Source: CAD feature listing. Evaluate the final solid. Frame: model axes, mm. A direction names the side the tool comes from. Coordinates: 2 decimals unless noted, no trailing zeros. Order: outer loops, then holes, each group sorted by start corner. A loop starts at its lowest first (then second) coordinate and runs counter-clockwise, first axis right, second up. Notation, with made-up numbers: (-37.75, 4.5) - (-15.75, 4.5) arc R34 ccw to (-15.75, 40.5) - close; hole circle Ø4 at (44.5, -28). An arc over 180 degrees is marked (long way). One line per question, with ' | ' between items.
from build123d import *

# Parameters (mm, degrees)
BOSS_EXTRUDE1_DEPTH      = 40
BOSS_EXTRUDE1_DEPTH_BACK = 10
SKETCH1_W                = 73
SKETCH1_H                = 3
SKETCH1_W_2              = 3
SKETCH1_H_2              = 10
SKETCH5_R                = 2.05
CUT_EXTRUDE2_DEPTH       = 5.1
CUT_EXTRUDE3_DEPTH       = 82
SKETCH9_W                = 50
SKETCH9_H                = 13
CUT_EXTRUDE4_DEPTH       = 0.5
CUT_EXTRUDE5_DEPTH       = 98.5
FILLET2_R                = 4
FILLET3_R                = 1


with BuildPart() as part:
    # Sketch1 → Boss-Extrude1 (new, two sides: drawn at the far end of the back side and taken through both)
    with BuildSketch(Plane.XY.offset(-BOSS_EXTRUDE1_DEPTH_BACK)):
        with Locations((0, -34)):
            Rectangle(SKETCH1_W, SKETCH1_H)
        with Locations((35, -40.5)):
            Rectangle(SKETCH1_W_2, SKETCH1_H_2)
        with Locations((-35, -40.5)):
            Rectangle(SKETCH1_W_2, SKETCH1_H_2)
    extrude(amount=BOSS_EXTRUDE1_DEPTH + BOSS_EXTRUDE1_DEPTH_BACK)

    # Sketch5 → Cut-Extrude2 (cut)
    with BuildSketch(Plane(origin=(0, -32.5, 0), x_dir=(1, 0, 0), z_dir=(0, 1, 0))):
        with Locations(Location((-19, 4, 0), (0, 0, 270))):
            Circle(SKETCH5_R)
        with Locations(Location((19, 4, 0), (0, 0, 270))):
            Circle(SKETCH5_R)
        with Locations(Location((19, -34, 0), (0, 0, 270))):
            Circle(SKETCH5_R)
        with Locations(Location((-19, -34, 0), (0, 0, 270))):
            Circle(SKETCH5_R)
        with BuildLine():
            Line((-31.5, -17), (-31.5, -13))
            ThreePointArc((-31.5, -13), (-30, -11.5), (-28.5, -13))
            Line((-28.5, -13), (-28.5, -17))
            ThreePointArc((-28.5, -17), (-30, -18.5), (-31.5, -17))
        make_face()
        with BuildLine():
            Line((31.5, -13), (31.5, -17))
            ThreePointArc((31.5, -17), (30, -18.5), (28.5, -17))
            Line((28.5, -17), (28.5, -13))
            ThreePointArc((28.5, -13), (30, -11.5), (31.5, -13))
        make_face()
    extrude(amount=-CUT_EXTRUDE2_DEPTH, mode=Mode.SUBTRACT)

    # Sketch8 → Cut-Extrude3 (cut)
    with BuildSketch(Plane.ZY.offset(36.5)):
        with BuildLine():
            Line((5.75, -38.4), (7.25, -38.4))
            ThreePointArc((7.25, -38.4), (8.85, -40), (7.25, -41.6))
            Line((7.25, -41.6), (5.75, -41.6))
            ThreePointArc((5.75, -41.6), (4.15, -40), (5.75, -38.4))
        make_face()
        with BuildLine():
            Line((24.25, -38.4), (22.75, -38.4))
            ThreePointArc((22.75, -38.4), (21.15, -40), (22.75, -41.6))
            Line((22.75, -41.6), (24.25, -41.6))
            ThreePointArc((24.25, -41.6), (25.85, -40), (24.25, -38.4))
        make_face()
    extrude(amount=-CUT_EXTRUDE3_DEPTH, mode=Mode.SUBTRACT)

    # Sketch9 → Cut-Extrude4 (cut)
    with BuildSketch(Plane.ZY.offset(36.5)):
        with Locations((15, -39)):
            Rectangle(SKETCH9_W, SKETCH9_H)
    cut_extrude4 = extrude(amount=-CUT_EXTRUDE4_DEPTH, mode=Mode.SUBTRACT)

    # Mirror1: Cut-Extrude4 across plane
    add(cut_extrude4.mirror(Plane(origin=(0, 0, 0), x_dir=(0, 0, 1), z_dir=(1, 0, 0))), mode=Mode.SUBTRACT)

    # Sketch10 → Cut-Extrude5 (cut)
    with BuildSketch(Plane(origin=(36, 0, 0), x_dir=(0, 0, -1), z_dir=(1, 0, 0))):
        with BuildLine():
            Line((-39.673112404, -45.5), (-40.667568966, -46.550213702))
            Line((-40.667568966, -46.550213702), (-44.63224415, -43))
            Line((-44.63224415, -43), (-42.018495325, -33.98072497))
            Line((-42.018495325, -33.98072497), (-39.463482429, -29.927945893))
            Line((-39.463482429, -29.927945893), (-37.524182533, -32.5))
            ThreePointArc((-37.524182533, -32.5), (-38.383444331, -36.355587887), (-39.532044935, -40.135085929))
            ThreePointArc((-39.532044935, -40.135085929), (-40.017082913, -42.806643803), (-39.673112404, -45.5))
        make_face()
    cut_extrude5 = extrude(amount=-CUT_EXTRUDE5_DEPTH, mode=Mode.SUBTRACT)

    # Fillet2
    # the kernel refuses this fillet: 4 mm, written as the material it takes off along each edge
    with BuildSketch(Plane(origin=(23.5, -45.5, -10), x_dir=(0, 1, 0), z_dir=(1, 0, 0)), Plane(origin=(-46, -45.5, -10), x_dir=(0, 1, 0), z_dir=(1, 0, 0))) as fillet2_piece_1:
        with BuildLine():
            CenterArc((FILLET2_R, FILLET2_R), FILLET2_R, 180, 90)
            Line((0, FILLET2_R), (-FILLET2_R * 0.02, FILLET2_R))
            Line((-FILLET2_R * 0.02, FILLET2_R), (-FILLET2_R * 0.02, -FILLET2_R * 0.02))
            Line((-FILLET2_R * 0.02, -FILLET2_R * 0.02), (FILLET2_R, -FILLET2_R * 0.02))
            Line((FILLET2_R, -FILLET2_R * 0.02), (FILLET2_R, 0))
        make_face()
    extrude(amount=22.5, mode=Mode.SUBTRACT)
    with BuildSketch(Plane(origin=(43.633505106, -45.5, 39.673112404), x_dir=(0, 0, -1), z_dir=(-1, 0, 0)), Plane(origin=(-25.866494894, -45.5, 39.673112404), x_dir=(0, 0, -1), z_dir=(-1, 0, 0))) as fillet2_piece_2:
        with BuildLine():
            CenterArc((3.053402042, -4), FILLET2_R, 90, 57.679694788)
            Line((-0.326887596, -1.861392518), (-0.394493388, -1.818620368))
            ThreePointArc((-0.394493388, -1.818620368), (-0.291841099, -0.908147826), (-0.076877032, 0.022134181))
            Line((-0.076877032, 0.022134181), (0, 0.08))
            Line((0, 0.08), (3.053402042, 0.08))
            Line((3.053402042, 0.08), (3.053402042, 0))
        make_face()
    extrude(amount=17.767010212, mode=Mode.SUBTRACT)

    # Mirror2: Cut-Extrude5 across plane
    add(cut_extrude5.mirror(Plane.XY.offset(15)), mode=Mode.SUBTRACT)

    # Fillet3
    # the kernel refuses this fillet: 1 mm, written as the material it takes off along each edge
    with BuildSketch(Plane(origin=(36, -43.040322305, -1.130093667), x_dir=(0, 0.32679600244698914, -0.9450949014700414), z_dir=(0, 0.9450949014700414, 0.32679600244698914))) as fillet3_piece_1:
        with BuildLine():
            CenterArc((8.890060939 - FILLET3_R, FILLET3_R), FILLET3_R, 270, 90)
            Line((8.890060939 - FILLET3_R, 0), (8.890060939 - FILLET3_R, -FILLET3_R * 0.02))
            Line((8.890060939 - FILLET3_R, -FILLET3_R * 0.02), (8.890060939 + FILLET3_R * 0.02, -FILLET3_R * 0.02))
            Line((8.890060939 + FILLET3_R * 0.02, -FILLET3_R * 0.02), (8.890060939 + FILLET3_R * 0.02, FILLET3_R))
            Line((8.890060939 + FILLET3_R * 0.02, FILLET3_R), (8.890060939, FILLET3_R))
        make_face()
    revolve(axis=Axis((36, -43.040322305, -1.130093667), (-1, 0, 0)), revolution_arc=51.275424055, mode=Mode.SUBTRACT)
    with BuildSketch(Plane(origin=(36, -43.040322305, 31.130093667), x_dir=(0, 0.32679600244698914, 0.9450949014700414), z_dir=(0, 0.9450949014700414, -0.32679600244698914))) as fillet3_piece_2:
        with BuildLine():
            CenterArc((8.890060939 - FILLET3_R, -FILLET3_R), FILLET3_R, 0, 90)
            Line((8.890060939 - FILLET3_R, 0), (8.890060939 - FILLET3_R, FILLET3_R * 0.02))
            Line((8.890060939 - FILLET3_R, FILLET3_R * 0.02), (8.890060939 + FILLET3_R * 0.02, FILLET3_R * 0.02))
            Line((8.890060939 + FILLET3_R * 0.02, FILLET3_R * 0.02), (8.890060939 + FILLET3_R * 0.02, -FILLET3_R))
            Line((8.890060939 + FILLET3_R * 0.02, -FILLET3_R), (8.890060939, -FILLET3_R))
        make_face()
    revolve(axis=Axis((36, -43.040322305, 31.130093667), (1, 0, 0)), revolution_arc=53.885597182, mode=Mode.SUBTRACT)
    with BuildSketch(Plane(origin=(-36, -43.040322305, -1.130093667), x_dir=(0, -0.532891092697407, -0.8461838354186183), z_dir=(0, -0.8461838354186183, 0.532891092697407))) as fillet3_piece_3:
        with BuildLine():
            CenterArc((8.890060939 - FILLET3_R, FILLET3_R), FILLET3_R, 270, 90)
            Line((8.890060939, FILLET3_R), (8.890060939 + FILLET3_R * 0.02, FILLET3_R))
            Line((8.890060939 + FILLET3_R * 0.02, FILLET3_R), (8.890060939 + FILLET3_R * 0.02, -FILLET3_R * 0.02))
            Line((8.890060939 + FILLET3_R * 0.02, -FILLET3_R * 0.02), (8.890060939 - FILLET3_R, -FILLET3_R * 0.02))
            Line((8.890060939 - FILLET3_R, -FILLET3_R * 0.02), (8.890060939 - FILLET3_R, 0))
        make_face()
    revolve(axis=Axis((-36, -43.040322305, -1.130093667), (1, 0, 0)), revolution_arc=51.275424055, mode=Mode.SUBTRACT)
    with BuildSketch(Plane(origin=(-36, -43.040322305, 31.130093667), x_dir=(0, 0.32679600244698914, 0.9450949014700414), z_dir=(0, 0.9450949014700414, -0.32679600244698914))) as fillet3_piece_4:
        with BuildLine():
            CenterArc((8.890060939 - FILLET3_R, FILLET3_R), FILLET3_R, 270, 90)
            Line((8.890060939 - FILLET3_R, 0), (8.890060939 - FILLET3_R, -FILLET3_R * 0.02))
            Line((8.890060939 - FILLET3_R, -FILLET3_R * 0.02), (8.890060939 + FILLET3_R * 0.02, -FILLET3_R * 0.02))
            Line((8.890060939 + FILLET3_R * 0.02, -FILLET3_R * 0.02), (8.890060939 + FILLET3_R * 0.02, FILLET3_R))
            Line((8.890060939 + FILLET3_R * 0.02, FILLET3_R), (8.890060939, FILLET3_R))
        make_face()
    revolve(axis=Axis((-36, -43.040322305, 31.130093667), (1, 0, 0)), revolution_arc=53.885597182, mode=Mode.SUBTRACT)
    with BuildSketch(Plane(origin=(36, -23.090673742, -58.824529959), x_dir=(0, -0.06631180934399998, 0.9977989496594617), z_dir=(0, 0.9977989496594617, 0.06631180934399998))) as fillet3_piece_5:
        with BuildLine():
            CenterArc((52.156122044 + FILLET3_R, -FILLET3_R), FILLET3_R, 90, 90)
            Line((52.156122044 + FILLET3_R, 0), (52.156122044 + FILLET3_R, FILLET3_R * 0.02))
            Line((52.156122044 + FILLET3_R, FILLET3_R * 0.02), (52.156122044 - FILLET3_R * 0.02, FILLET3_R * 0.02))
            Line((52.156122044 - FILLET3_R * 0.02, FILLET3_R * 0.02), (52.156122044 - FILLET3_R * 0.02, -FILLET3_R))
            Line((52.156122044 - FILLET3_R * 0.02, -FILLET3_R), (52.156122044, -FILLET3_R))
        make_face()
    revolve(axis=Axis((36, -23.090673742, -58.824529959), (1, 0, 0)), revolution_arc=15.272244004, mode=Mode.SUBTRACT)
    with BuildSketch(Plane(origin=(36, -23.090673742, 88.824529959), x_dir=(0, -0.06631180934399998, -0.9977989496594617), z_dir=(0, 0.9977989496594617, -0.06631180934399998))) as fillet3_piece_6:
        with BuildLine():
            CenterArc((52.156122044 + FILLET3_R, FILLET3_R), FILLET3_R, 180, 90)
            Line((52.156122044 + FILLET3_R, 0), (52.156122044 + FILLET3_R, -FILLET3_R * 0.02))
            Line((52.156122044 + FILLET3_R, -FILLET3_R * 0.02), (52.156122044 - FILLET3_R * 0.02, -FILLET3_R * 0.02))
            Line((52.156122044 - FILLET3_R * 0.02, -FILLET3_R * 0.02), (52.156122044 - FILLET3_R * 0.02, FILLET3_R))
            Line((52.156122044 - FILLET3_R * 0.02, FILLET3_R), (52.156122044, FILLET3_R))
        make_face()
    revolve(axis=Axis((36, -23.090673742, 88.824529959), (-1, 0, 0)), revolution_arc=15.272244004, mode=Mode.SUBTRACT)
    with BuildSketch(Plane(origin=(-36, -23.090673742, -58.824529959), x_dir=(0, -0.06631180934399998, 0.9977989496594617), z_dir=(0, 0.9977989496594617, 0.06631180934399998))) as fillet3_piece_7:
        with BuildLine():
            CenterArc((52.156122044 + FILLET3_R, FILLET3_R), FILLET3_R, 180, 90)
            Line((52.156122044 + FILLET3_R, 0), (52.156122044 + FILLET3_R, -FILLET3_R * 0.02))
            Line((52.156122044 + FILLET3_R, -FILLET3_R * 0.02), (52.156122044 - FILLET3_R * 0.02, -FILLET3_R * 0.02))
            Line((52.156122044 - FILLET3_R * 0.02, -FILLET3_R * 0.02), (52.156122044 - FILLET3_R * 0.02, FILLET3_R))
            Line((52.156122044 - FILLET3_R * 0.02, FILLET3_R), (52.156122044, FILLET3_R))
        make_face()
    revolve(axis=Axis((-36, -23.090673742, -58.824529959), (1, 0, 0)), revolution_arc=15.272244004, mode=Mode.SUBTRACT)
    with BuildSketch(Plane(origin=(-36, -23.090673742, 88.824529959), x_dir=(0, -0.32679600244698953, -0.9450949014700414), z_dir=(0, -0.9450949014700414, 0.32679600244698953))) as fillet3_piece_8:
        with BuildLine():
            CenterArc((52.156122044 + FILLET3_R, FILLET3_R), FILLET3_R, 180, 90)
            Line((52.156122044 + FILLET3_R, 0), (52.156122044 + FILLET3_R, -FILLET3_R * 0.02))
            Line((52.156122044 + FILLET3_R, -FILLET3_R * 0.02), (52.156122044 - FILLET3_R * 0.02, -FILLET3_R * 0.02))
            Line((52.156122044 - FILLET3_R * 0.02, -FILLET3_R * 0.02), (52.156122044 - FILLET3_R * 0.02, FILLET3_R))
            Line((52.156122044 - FILLET3_R * 0.02, FILLET3_R), (52.156122044, FILLET3_R))
        make_face()
    revolve(axis=Axis((-36, -23.090673742, 88.824529959), (1, 0, 0)), revolution_arc=15.272244004, mode=Mode.SUBTRACT)


solid = part.part
(1) Set-up query: faces 1 (the flat face through (-35, -38.4, 6)), 2 (the cylindrical face through (-30, -34, 18.5)), 3 (the flat face through (0, -35.5, 15)). Return all of +Z, -Z, +X, -X, +Y, -Y with unobstructed straight access to the full face (end or side cutting, diameter ignored); none if empty.
Taken from the geometry:
face 1: +X, -X | face 2: +Y, -Y | face 3: +Z, -Z, -Y
(2) Pull-direction query (X, two-part tool) for faces 4 (the cylindrical face through (20.4, -34, -5.5)), 5 (the cylindrical face through (34.73, -39.96, 21.15)), 6 (the flat face through (33.5, -41, 15)); classes: pulls with the +X half, pulls with the -X half, needs draft (parallel to the pull), parting line crosses it, or undercut.
Taken from the geometry:
face 4: undercut | face 5: needs draft | face 6: undercut
(3) Pin query (flat end, axial travel): P1, Ø1.5, axis at x = -9.5, y = -35.5, coming from the +Z side; P2, Ø3, axis at x = -22, z = 16.5, coming from the -Y side; P3, Ø3, axis at x = 27, y = -35, coming from the -Z side; P4, Ø3.5, axis at x = 19, z = 34, coming from the +Y side. Return the tip coordinate at first contact, or that it passes through.
Taken from the geometry:
P1: stops at z = 38.17 | P2: stops at y = -35.5 | P3: stops at z = -8.17 | P4: passes through
(4) Material intervals for L1, parallel to X at y = -34.55, z = -4; L2, parallel to X at y = -39.75, z = 0; L3, parallel to Y at x = 26, z = 23.5, sorted ascending. Write a range as from..to.
Taken from the geometry:
L1: x = -36..-21.05, -16.95..16.95, 21.05..36 | L2: x = -36..-33.5, 33.5..36 | L3: y = -35.5..-32.5
(5) Cut plane B-B (x = -30). Return the cut outline in (y, z).
Taken from the geometry:
outline: (-35.5, -8.17) arc R52.16 cw to (-32.5, -7.52) - (-32.5, 11.5) - (-35.5, 11.5) - close; (-35.5, 18.5) - (-32.5, 18.5) - (-32.5, 37.52) arc R52.16 cw to (-35.5, 38.17) - close
(6) Cut plane D-D (z = -4). Return the cut outline in (x, y).
Taken from the geometry:
outline: (-36, -45.5) - (-33.5, -45.5) - (-33.5, -35.5) - (-21.05, -35.5) - (-21.05, -32.5) - (-36, -32.5) - close; (-16.95, -35.5) - (16.95, -35.5) - (16.95, -32.5) - (-16.95, -32.5) - close; (21.05, -35.5) - (33.5, -35.5) - (33.5, -45.5) - (36, -45.5) - (36, -32.5) - (21.05, -32.5) - close
(7) Cut plane A-A (z = 23.5). Return the cut outline in (x, y).
Taken from the geometry:
outline: (-36, -45.5) - (-33.5, -45.5) - (-33.5, -41.6) - (-36, -41.6) - close; (-36, -38.4) - (-33.5, -38.4) - (-33.5, -35.5) - (33.5, -35.5) - (33.5, -38.4) - (36, -38.4) - (36, -32.5) - (-36, -32.5) - close; (33.5, -45.5) - (36, -45.5) - (36, -41.6) - (33.5, -41.6) - close
(8) Cut plane C-C (z = 1.5). Return the cut outline in (x, y), and give its area (3 significant figures).
Taken from the geometry:
outline: (-36, -45.5) - (-33.5, -45.5) - (-33.5, -35.5) - (33.5, -35.5) - (33.5, -45.5) - (36, -45.5) - (36, -32.5) - (-36, -32.5) - close | area: 266 mm²
